Can you work these out from the model? Positions are in its coordinate system, mm. A direction names the side the tool comes from. Coordinates: 2 decimals unless noted, no trailing zeros. Order: outer loops, then holes, each group sorted by start corner. A loop starts at its lowest first (then second) coordinate and runs counter-clockwise, first axis right, second up. Notation, with made-up numbers: (27, 26) -> (34, 26) arc R10 cw to (34, 38) -> close; hole circle Ø6 at (31, 1.5). An arc over 180 degrees is marked (long way). Answer as a JSON object with one key per item and string values. Group by question number.
(1) For pin 1 (1 mm diameter, centred on x = 242, y = 5, fed in from -Z), with a flat end and sliding along its axis, tell me the tip position at first contact or that it passes through.
(2) I want a section at B-B, the plane x = 603.5. List the corners of the cut face in (y, z) for me.
(3) If we mould it in two halves opening along X, with no side actions, what happens to faces 1 (the flat face through (493, 0, -557)), 2 (the flat face through (452, 14, -536)), 3 (the flat face through (0, 14, -296))? For each: pulls with the +X half, pulls with the -X half, needs draft (parallel to the pull), parting line crosses it, or undercut.
(4) Which directions (+Z, -Z, +X, -X, +Y, -Y) give clear straight access to the entire face, cutting with the end or side of a thin tool? Please do faces 4 (the flat face through (174.938, 14, -287)), 5 (the flat face through (1000, 14, -296)).
(5) I need wall thicknesses on line 1 (X direction, y = 19, z = -259.5); line 2 (Z direction, x = 208, y = 13.25); line 3 (Z direction, x = 218, y = 23.75). Which ranges of each line are inside material? Lowest first, please.
(6) I want a section at A-A, the plane z = -297. List the corners of the cut face in (x, y) for me, plus the area to 3 significant figures.
(7) I want a section at C-C, the plane y = 15.25. List the corners of the cut face in (x, z) for me, plus the area to 3 significant figures.
from build123d import *

# Parameters (mm, degrees)
EXTRUDE_1_DEPTH     = 1000
SKETCH_3_W          = 561
SKETCH_3_H          = 491
CUT_EXTRUDE_1_DEPTH = 29


with BuildPart() as part:
    # Эскиз2 → Бобышка-Вытянуть1 (new body)
    with BuildSketch(Plane(origin=(0, 0, 0), x_dir=(0, 0, -1), z_dir=(1, 0, 0))):
        with BuildLine():
            Line((0, 0), (594, 0))
            ThreePointArc((594, 0), (598.242640687, 1.757359313), (600, 6))
            Line((600, 6), (600, 22))
            ThreePointArc((600, 22), (598.242640687, 26.242640687), (594, 28))
            Line((594, 28), (0, 28))
            Line((0, 28), (0, 0))
        make_face()
    extrude(amount=EXTRUDE_1_DEPTH)

    # Эскиз3 → Вырез-Вытянуть1 (cut, through all)
    with BuildSketch(Plane(origin=(0, 28, 0), x_dir=(1, 0, 0), z_dir=(0, 1, 0))):
        with Locations((455.438358963, 290.5)):
            Rectangle(SKETCH_3_W, SKETCH_3_H)
    extrude(amount=-CUT_EXTRUDE_1_DEPTH, mode=Mode.SUBTRACT)


solid = part.part
Computed values:
{
 "1": {"pin 1": "stops at z = -599.98"},
 "2": {"outline": "(0, -594) arc R6 ccw to (6, -600) -> (22, -600) arc R6 ccw to (28, -594) -> (28, -536) -> (0, -536) -> close; (0, -45) -> (28, -45) -> (28, 0) -> (0, 0) -> close"},
 "3": {"face 1": "needs draft", "face 2": "undercut", "face 3": "pulls with the -X half"},
 "4": {"face 4": "+Y, -Y", "face 5": "+Z, -Z, +X, +Y, -Y"},
 "5": {"line 1": "x = 0 to 174.94, 735.94 to 1000", "line 2": "z = -600 to -536, -45 to 0", "line 3": "z = -599.74 to -536, -45 to 0"},
 "6": {"outline": "(0, 0) -> (174.94, 0) -> (174.94, 28) -> (0, 28) -> close; (735.94, 0) -> (1000, 0) -> (1000, 28) -> (735.94, 28) -> close", "area": "12,300 mm2"},
 "7": {"outline": "(0, -600) -> (1000, -600) -> (1000, 0) -> (0, 0) -> close; hole (174.94, -536) -> (735.94, -536) -> (735.94, -45) -> (174.94, -45) -> close", "area": "325,000 mm2"}
}
